The listing builds one solid part. Answer for the finished solid, in the listing's coordinates (mm). A direction names the side the tool comes from. Round coordinates to 2 decimals unless told otherwise and drop trailing zeros. Write each loop counter-clockwise with the first axis right and the second up, starting at its lowest first coordinate (ties: lowest second). Pieces come first, ordered by that corner, then holes.
from build123d import *

# Parameters (mm, degrees)
BOSS_EXTRUDE1_DEPTH     = 9
FILLET1_R               = 2
CUT_EXTRUDE1_DEPTH      = 38.496666519
CUT_EXTRUDE1_DEPTH_BACK = 38.496666519
SKETCH3_R               = 2.5
BOSS_EXTRUDE2_DEPTH     = 10
CUT_EXTRUDE2_DEPTH      = 42.303752856
CUT_EXTRUDE2_DEPTH_BACK = 42.303752856
SKETCH4_R               = 0.75
SKETCH5_W               = 1
SKETCH5_H               = 10
BOSS_EXTRUDE3_DEPTH     = 10


with BuildPart() as part:
    # Sketch1 → Boss-Extrude1 (new, symmetric)
    with BuildSketch(Plane.XY):
        with BuildLine():
            ThreePointArc((-33.714795211, -0.491812162), (-34.647663561, 0.242423764), (-35, 1.376092494))
            Line((-35, 1.376092494), (-35, 10))
            Line((-35, 10), (35, 10))
            Line((35, 10), (35, 1.330500849))
            ThreePointArc((35, 1.330500849), (34.665188238, 0.222733667), (33.772851869, -0.514140034))
            Line((33.772851869, -0.514140034), (11.50283608, -9.844640883))
            ThreePointArc((11.50283608, -9.844640883), (11.12414042, -9.960775582), (10.729984211, -10))
            Line((10.729984211, -10), (-8.498371341, -10))
            ThreePointArc((-8.498371341, -10), (-8.861820571, -9.966698924), (-9.213166552, -9.867904657))
            Line((-9.213166552, -9.867904657), (-33.714795211, -0.491812162))
        make_face()
    extrude(amount=BOSS_EXTRUDE1_DEPTH, both=True)

    # Fillet1
    fillet1_edges = [part.edges().sort_by_distance(p)[0] for p in [
        (0, 10, -9),
        (0, 10, 9),
    ]]
    fillet(fillet1_edges, radius=FILLET1_R)

    # Sketch2 → Cut-Extrude1 (cut, two sides: drawn at the far end of the back side and taken through both)
    with BuildSketch(Plane(origin=(0, 0, 0), x_dir=(0, 0, -1), z_dir=(1, 0, 0)).offset(-CUT_EXTRUDE1_DEPTH_BACK)):
        with BuildLine():
            Line((-8, 8), (-8, -14.234256749))
            Line((-8, -14.234256749), (8, -14.234256749))
            Line((8, -14.234256749), (8, 1.330500849))
            Line((8, 1.330500849), (8, 8))
            ThreePointArc((8, 8), (7.707106781, 8.707106781), (7, 9))
            Line((7, 9), (-7, 9))
            ThreePointArc((-7, 9), (-7.707106781, 8.707106781), (-8, 8))
        make_face()
    extrude(amount=CUT_EXTRUDE1_DEPTH + CUT_EXTRUDE1_DEPTH_BACK, mode=Mode.SUBTRACT)

    # Sketch3 → Boss-Extrude2 (add)
    with BuildSketch(Plane(origin=(0, 10, 0), x_dir=(1, 0, 0), z_dir=(0, 1, 0))):
        with Locations(Location((0, 0, 0), (0, 0, 270))):
            Circle(SKETCH3_R)
    extrude(amount=BOSS_EXTRUDE2_DEPTH)

    # Sketch4 → Cut-Extrude2 (cut, two sides: drawn at the far end of the back side and taken through both)
    with BuildSketch(Plane.XY.offset(-CUT_EXTRUDE2_DEPTH_BACK)):
        with Locations((-30, 2)):
            Circle(SKETCH4_R)
        with Locations((-22, 2)):
            Circle(SKETCH4_R)
        with Locations((-5, -5)):
            Circle(SKETCH4_R)
        with Locations(Location((5, -5, 0), (0, 0, 180))):
            Circle(SKETCH4_R)
        with Locations(Location((22, 2, 0), (0, 0, 180))):
            Circle(SKETCH4_R)
        with Locations(Location((30, 2, 0), (0, 0, 180))):
            Circle(SKETCH4_R)
    extrude(amount=CUT_EXTRUDE2_DEPTH + CUT_EXTRUDE2_DEPTH_BACK, mode=Mode.SUBTRACT)

    # Sketch5 → Boss-Extrude3 (add)
    with BuildSketch(Plane.XZ.offset(-9)):
        with Locations((0.5, 0)):
            Rectangle(SKETCH5_W, SKETCH5_H)
    extrude(amount=BOSS_EXTRUDE3_DEPTH)


solid = part.part
1. For a pull along X with two mould halves and no side action, classify faces 1 (the face through (-35, 9.2, 1.4)), 2 (the face through (22.75, 1.97, -8.51)), 3 (the face through (35, 9.2, 1.4)), 4 (the face through (0, 20, 0)) as released by +X, released by -X, zero draft, split by the parting line, or undercut.
Geometry says:
face 1: released by -X
face 2: undercut
face 3: released by +X
face 4: zero draft
2. Section D-D on y = -7.5 is taken. Determine the outline of the cut face in (x, z).
Geometry says:
outline: (-15.4, -9) - (17.1, -9) - (17.1, -8) - (-15.4, -8) - close; (-15.4, 8) - (17.1, 8) - (17.1, 9) - (-15.4, 9) - close
3. Section B-B on x = 30 is taken. Determine the outline of the cut face in (y, z).
Geometry says:
outline: (-2.09, -9) - (1.25, -9) - (1.25, -8) - (-2.09, -8) - close; (-2.09, 8) - (1.25, 8) - (1.25, 9) - (-2.09, 9) - close; (2.75, -9) - (8, -9) arc R2 ccw to (10, -7) - (10, 7) arc R2 ccw to (8, 9) - (2.75, 9) - (2.75, 8) - (8, 8) arc R1 cw to (9, 7) - (9, -7) arc R1 cw to (8, -8) - (2.75, -8) - close
4. Given pin 1 (4 mm diameter, centred on x = -4.5, z = 0, fed in from -Y); pin 2 (8 mm diameter, centred on y = -0.5, z = 0.5, fed in from -X); pin 3 (0.5 mm diameter, centred on x = 0.5, z = 0.5, fed in from -Y); pin 4 (0.9 mm diameter, centred on x = 5, y = -5, fed in from -Z), each flat-ended and moving along its own axis, determine where each tip first touches the part or whether it passes through.
Geometry says:
pin 1: stops at y = 9
pin 2: stops at x = 0
pin 3: stops at y = -1
pin 4: passes through
5. Straight lines are drawn through the part: line 1 along Z through (x, y) = (13, 4.75); line 2 along Y through (x, z) = (13, 0.5); line 3 along Y through (x, z) = (30, 8.8). For each, find the intervals that lie inside material, in ascending order.
Geometry says:
line 1: z = -9 to -8, 8 to 9
line 2: y = 9 to 10
line 3: y = -2.09 to 1.25, 2.75 to 8.87
6. Section C-C on z = 3.5 is taken. Determine the outline of the cut face in (x, y), plus the area to 3 significant figures.
Geometry says:
outline: (-35, 9) - (0, 9) - (0, -1) - (1, -1) - (1, 9) - (35, 9) - (35, 10) - (-35, 10) - close
area: 80.0 mm2
7. Section A-A on y = 4.5 is taken. Determine the outline of the cut face in (x, z), plus the area to 3 significant figures.
Geometry says:
outline: (-35, -9) - (35, -9) - (35, -8) - (-35, -8) - close; (-35, 8) - (35, 8) - (35, 9) - (-35, 9) - close; (0, -5) - (1, -5) - (1, 5) - (0, 5) - close
area: 150 mm2
8. A tool of negligible diameter and unlimited length cuts with its end or side. For faces 5 (the face through (0, 1, 8)), 6 (the face through (5.595, -4.544, -8.507)), from which of +Z, -Z, +X, -X, +Y, -Y can it reach the whole face along a straight path? Write none if from no direction.
Geometry says:
face 5: +X, -X, -Y
face 6: +Z, -Z
